Verification items for this drawing (mm, ordinates from the low corner). Give positions to 0.01 mm unless a question says otherwise; leave off trailing zeros. Order: outer loops, then holes, each group sorted by start corner. A loop starts at its lowest first (then second) coordinate and runs counter-clockwise, first axis right, second up. Notation, with made-up numbers: M 0,81.5 L 37,81.5 A11 ccw 37,95.5 Z; hole C -33,-9 d4. An arc over 180 degrees is marked long. Return JSON: item names as keys, results as strings. Group by question number.
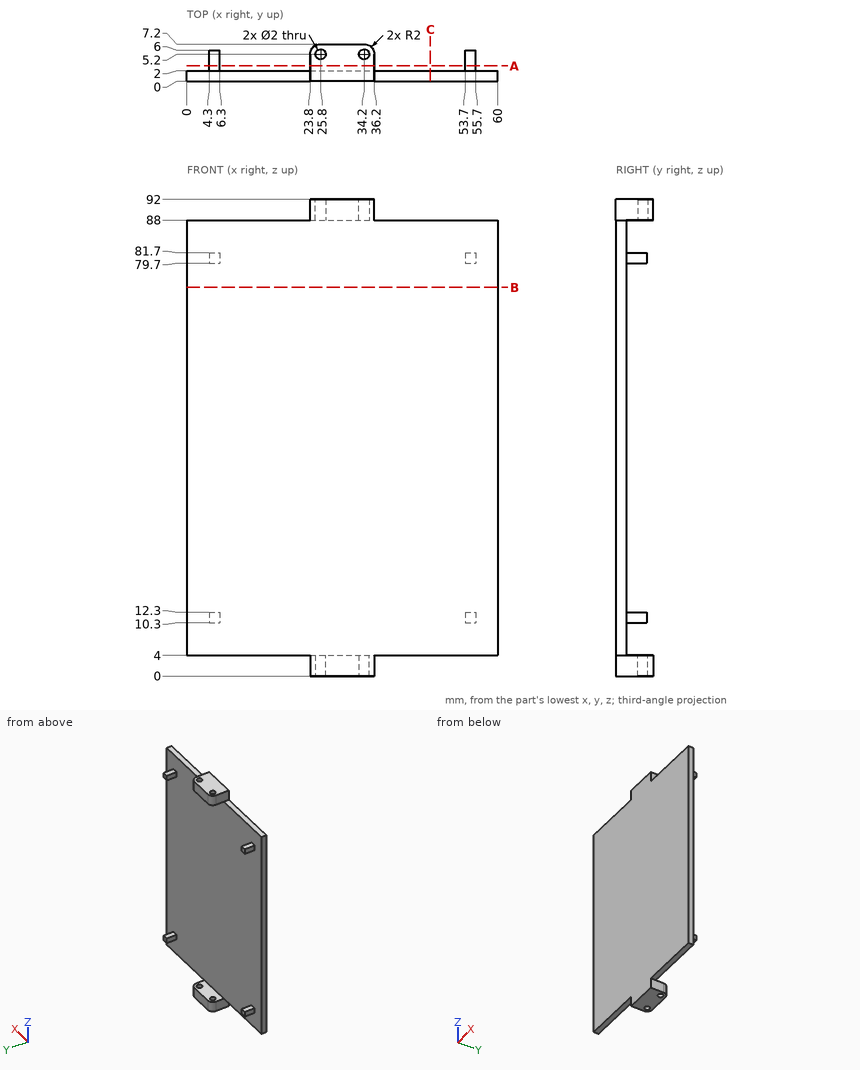
1) Sectioned sample at B-B on z = 75. Record the boundary of the cut face in (x, y), then the cut area to 3 significant figures.
2) Sectioned sample at C-C on x = 47. Record the boundary of the cut face in (y, z).
3) Sectioned sample at A-A on y = 3. Record the boundary of the cut face in (x, z).
4) Material ranges on line 1 along Y through (x, z) = (25.8, 0.95); line 2 along Y through (x, z) = (37.5, 73); line 3 along Z through (x, y) = (30, 3), recorded low to high.
5) Depth check by flat-ended pin: P1, Ø2, axis at x = 38.5, z = 26.5, coming from the +Y side; P2, Ø1, axis at x = 55, z = 12, coming from the +Y side; P3, Ø4, axis at x = 21.5, y = 6, coming from the +Z side; P4, Ø2, axis at x = 54.5, y = 3.5, coming from the +Z side. Enter the tip coordinate at first touch or a pass-through.
Reply:
{
 "1": {"outline": "M 0,0 L 60,0 L 60,2 L 0,2 Z", "area": "120 mm^2"},
 "2": {"outline": "M 0,4 L 2,4 L 2,88 L 0,88 Z"},
 "3": {"outline": "M 4.3,10.3 L 6.3,10.3 L 6.3,12.3 L 4.3,12.3 Z; M 4.3,79.7 L 6.3,79.7 L 6.3,81.7 L 4.3,81.7 Z; M 23.8,0 L 36.2,0 L 36.2,4 L 23.8,4 Z; M 23.8,88 L 36.2,88 L 36.2,92 L 23.8,92 Z; M 53.7,10.3 L 55.7,10.3 L 55.7,12.3 L 53.7,12.3 Z; M 53.7,79.7 L 55.7,79.7 L 55.7,81.7 L 53.7,81.7 Z"},
 "4": {"line 1": "0 to 4.2, 6.2 to 7.2", "line 2": "0 to 2", "line 3": "0 to 4, 88 to 92"},
 "5": {"P1": "y = 2", "P2": "y = 6", "P3": "through", "P4": "z = 81.7"}
}
